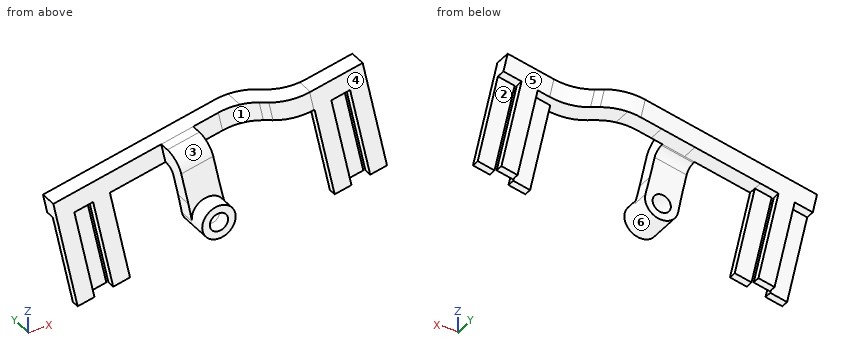
```python
from build123d import *

# Parameters (mm, degrees)
SKETCH1_R             = 3.175
BOSS_EXTRUDE1_DEPTH   = 8.89
F_4_CLEARANCE_HOLE1_D = 3.4544
BOSS_EXTRUDE2_START   = -3.175
BOSS_EXTRUDE2_DEPTH   = 3.175
BOSS_EXTRUDE3_DEPTH   = 3.81
BOSS_EXTRUDE4_START   = -9.525
BOSS_EXTRUDE4_DEPTH   = 3.175
CUT_EXTRUDE1_DEPTH    = 18.185920344
CUT_EXTRUDE2_DEPTH    = 5.08
BOSS_EXTRUDE5_START   = -20.938172
BOSS_EXTRUDE5_DEPTH   = 6.208698
BOSS_EXTRUDE6_DEPTH   = 3.175
FILLET2_R             = 8.89
FILLET3_R             = 1.5875
FILLET4_R             = 3.175
SKETCH16_R            = 3.175
SKETCH16_R_2          = 1.7272
BOSS_EXTRUDE7_DEPTH   = 2.54


with BuildPart() as part:
    # Sketch1 → Boss-Extrude1 (new body)
    with BuildSketch(Plane(origin=(0, 0, 0), x_dir=(1, 0, 0), z_dir=(0, 1, 0))):
        with Locations(Location((0, 0, 0), (0, 0, 270))):
            Circle(SKETCH1_R)
    extrude(amount=BOSS_EXTRUDE1_DEPTH)

    # #4 Clearance Hole1 (through all)
    with Locations(Plane(origin=(0, 8.89, 0), x_dir=(1, 0, 0), z_dir=(0, 1, 0))):
        with Locations((0, 0)):
            Hole(F_4_CLEARANCE_HOLE1_D / 2)

    # Sketch5 → Boss-Extrude2 (add)
    with BuildSketch(Plane(origin=(0, 8.89, 0), x_dir=(1, 0, 0), z_dir=(0, 1, 0)).offset(BOSS_EXTRUDE2_START)):
        with BuildLine():
            Line((-26.325590973, -8.090556636), (8.584422353, -15.580785179))
            Line((8.584422353, -15.580785179), (9.383698549, -11.85556605))
            Line((9.383698549, -11.85556605), (3.175, -10.523439056))
            Line((3.175, -10.523439056), (3.175, 0))
            ThreePointArc((3.175, 0), (0, -3.175), (-3.175, 0))
            Line((-3.175, 0), (-3.175, -9.160994683))
            Line((-3.175, -9.160994683), (-15.592397098, -6.496740696))
            Line((-15.592397098, -6.496740696), (-11.777286014, 11.284502966))
            Line((-11.777286014, 11.284502966), (-21.711203692, 13.415906155))
            Line((-21.711203692, 13.415906155), (-26.325590973, -8.090556636))
        make_face()
    extrude(amount=BOSS_EXTRUDE2_DEPTH)

    # Sketch11 → Boss-Extrude3 (add)
    with BuildSketch(Plane(origin=(-2.818068695, 0, 13.134287577), x_dir=(0.977747803012258, 0, 0.20978377845940036), z_dir=(-0.20978377845940033, 0, 0.9777478030122579))):
        Polygon((11.661996082, 8.89), (12.977124143, 8.89), (19.327124143, 2.54), (21.821996082, 2.54), (21.821996082, -0.635), (18.011996082, -0.635), (11.661996082, 5.715), align=None)
    extrude(amount=-BOSS_EXTRUDE3_DEPTH)

    # Sketch12 → Boss-Extrude4 (add)
    with BuildSketch(Plane(origin=(0, 8.89, 0), x_dir=(1, 0, 0), z_dir=(0, 1, 0)).offset(BOSS_EXTRUDE4_START)):
        Polygon((18.518340032, -17.712188368), (23.132727312, 3.794274423), (33.066644991, 1.662871234), (28.45225771, -19.843591557), align=None)
    extrude(amount=BOSS_EXTRUDE4_DEPTH)

    # Sketch6 → Cut-Extrude1 (cut)
    with BuildSketch(Plane(origin=(1.796318586, 0, -8.372175215), x_dir=(-0.977747803012258, 0, -0.20978377845940016), z_dir=(0.20978377845940016, 0, -0.977747803012258))):
        Polygon((17.142187862, 7.1755), (17.142187862, 5.715), (20.782854529, 5.715), (20.782854529, 7.1755), (24.042521196, 7.1755), (24.042521196, 8.89), (20.528854529, 8.89), (20.528854529, 7.4295), (17.396187862, 7.4295), (17.396187862, 8.89), (13.882521196, 8.89), (13.882521196, 7.1755), align=None)
        Polygon((-28.722329416, 0.8255), (-28.722329416, -0.635), (-25.081662749, -0.635), (-25.081662749, 0.8255), (-21.821996082, 0.8255), (-21.821996082, 2.54), (-25.335662749, 2.54), (-25.335662749, 1.0795), (-28.468329416, 1.0795), (-28.468329416, 2.54), (-31.981996082, 2.54), (-31.981996082, 0.8255), align=None)
    extrude(amount=-CUT_EXTRUDE1_DEPTH, mode=Mode.SUBTRACT)

    # Sketch13 → Cut-Extrude2 (cut)
    with BuildSketch(Plane(origin=(0, 8.89, 0), x_dir=(1, 0, 0), z_dir=(0, 1, 0))):
        Polygon((-3.175, -9.160994683), (3.175, -10.523439056), (3.175, 7.256560944), (-3.175, 7.256560944), align=None)
    extrude(amount=-CUT_EXTRUDE2_DEPTH, mode=Mode.SUBTRACT)


with BuildPart() as cut_extrude2_piece_1:
    # of the separate pieces the step leaves, piece 1, a body of its own (cut_extrude2_pieces)
    add(part.part.solids().sort_by_distance((-18.52407177, 5.715, -12.732080965))[0])

    # Sketch14 → Boss-Extrude5 (add)
    with BuildSketch(Plane(origin=(-23.507522278, 0, -5.04373094), x_dir=(-0.20978377845940016, 0, 0.977747803012258), z_dir=(-0.977747803012258, 0, -0.20978377845940016)).offset(BOSS_EXTRUDE5_START)):
        Polygon((3.81, 0.635), (13.433205921, 0.635), (13.433205921, 5.715), (9.635481661, 5.715), (9.623205921, 5.715), (9.623205921, 3.81), (3.81, 3.81), align=None)
    extrude(amount=-BOSS_EXTRUDE5_DEPTH)



with BuildPart() as cut_extrude2_piece_2:
    # of the separate pieces the step leaves, piece 2, a body of its own (cut_extrude2_pieces)
    add(part.part.solids().sort_by_distance((0, 0, 3.175))[0])


with BuildPart() as cut_extrude2_piece_1_1:
    add(cut_extrude2_piece_1.part)

    add(cut_extrude2_piece_2.part)  # Boss-Extrude6 merges Cut-Extrude2 piece 2
    # Sketch15 → Boss-Extrude6 (add)
    with BuildSketch(Plane(origin=(0, 3.81, 0), x_dir=(1, 0, 0), z_dir=(0, 1, 0))):
        with BuildLine():
            Line((-3.834546879, -3.073977009), (-3.116253173, 0.607940096))
            ThreePointArc((-3.116253173, 0.607940096), (-0.666063497, -3.104349275), (3.091361375, -0.723954316))
            Line((3.091361375, -0.723954316), (2.235994487, -4.37646125))
            Line((2.235994487, -4.37646125), (-3.834546879, -3.073977009))
        make_face()
    extrude(amount=-BOSS_EXTRUDE6_DEPTH)

    # Fillet2
    fillet2_edges = [cut_extrude2_piece_1_1.edges().sort_by_distance(p)[0] for p in [
        (8.984060451, 5.715, 13.718175614),
        (10.269924023, 8.89, 13.994068148),
        (16.478622572, 2.54, 15.326195141),
        (15.192759, -0.635, 15.050302607),
    ]]
    fillet(fillet2_edges, radius=FILLET2_R)

    # Fillet3
    fillet3_edges = [cut_extrude2_piece_1_1.edges().sort_by_distance(p)[0] for p in [
        (-2.01879269, 3.81, 9.409068406),
    ]]
    fillet(fillet3_edges, radius=FILLET3_R)

    # Fillet4
    fillet4_edges = [cut_extrude2_piece_1_1.edges().sort_by_distance(p)[0] for p in [
        (-2.818068886, 0.635, 13.134287535),
    ]]
    fillet(fillet4_edges, radius=FILLET4_R)

    # Sketch16 → Boss-Extrude7 (add)
    with BuildSketch(Plane.XZ):
        with Locations(Location((0, 0, 0), (0, 0, 270))):
            Circle(SKETCH16_R)
        with Locations(Location((0, 0, 0), (0, 0, 270))):
            Circle(SKETCH16_R_2, mode=Mode.SUBTRACT)
    extrude(amount=BOSS_EXTRUDE7_DEPTH)


solid = cut_extrude2_piece_1_1.part
```
The model under review builds one solid part; all positions refer to its coordinate system, in mm. Face numbers are marked on the shaded views. A direction names the side the tool comes from. Round coordinates to 2 decimals unless told otherwise and drop trailing zeros. Loops run counter-clockwise (first coordinate to the right, second up) from the corner with the lowest first, then second, coordinate; pieces in that order, holes last. Notation, with made-up numbers: (33.25, -13) - (90.25, -13) arc R11 ccw to (90.25, -6) - close; hole circle Ø2 at (81.5, 51). An arc over 180 degrees is marked (long way). Write each question's results on one line, items separated by ' | '. Start each with the question number.
Q1. Insertion check: P1, Ø10, axis at x = 19.5, z = 7.5, coming from the -Y side (3 decimals); P2, Ø8, axis at x = 24, z = 10.5, coming from the +Y side; P3, Ø5.5, axis at x = -23, z = -5.5, coming from the +Y side; P4, Ø4.5, axis at x = 0, z = 0, coming from the -Y side. Each pin has a flat end and moves straight along its axis. Give the tip position at first contact, or say it passes through.
Q2. Wall thickness on line 1 along X through (y, z) = (-0.9, 0) (3 decimals); line 2 along X through (y, z) = (1.25, 0.5); line 3 along Z through (x, y) = (0, 2.2) (3 decimals): over which ranges is each line inside the solid? List them lowest first. Write a range as [from, to].
Q3. Take a section at C-C on y = 8. Give the boundary of the cut face in (x, z) (3 decimals), plus the area to 3 significant figures.
Q4. Tool access review of the marked faces 4, 5 and 6: name each direction out of +Z, -Z, +X, -X, +Y, -Y from which nothing blocks a thin tool from reaching the whole face with its end or side.
Q5. Take a section at B-B on z = 0. Give the number of separate pieces and of enclosed holes in the cut face, plus the area to 3 significant figures.
Q6. Take a section at A-A on z = -6. Give the boundary of the cut face in (x, y) (1 decimal).
Q7. Draft analysis for pull direction X (two halves, no side actions). For the marked faces 1, 2 and 3, state which applies: pulls with the +X half, pulls with the -X half, needs draft (parallel to the pull), parting line crosses it, or undercut.
Data:
1) P1: stops at y = -0.635 | P2: stops at y = 2.54 | P3: stops at y = 7.18 | P4: stops at y = -2.54
2) line 1: x = [-3.175, -1.727], [1.727, 3.175] | line 2: x = [-3.33, -1.65], [1.65, 3.14], [25.8, 29.01] | line 3: z = [-3.175, -1.727], [1.727, 13.29]
3) outline: (-26.326, 8.091) - (-25.526, 4.365) - (-22.091, 5.102) - (-18.276, -12.679) - (-15.213, -12.022) - (-19.028, 5.76) - (10.86, 12.172) - (10.061, 15.898) - close | area: 199 mm²
4) face 4: +Z, -Z, +X, -Y | face 5: +Z, -Z, +X, +Y | face 6: -Y
5) separate pieces: 8 | enclosed holes: 0 | area: 47.4 mm²
6) outline: (-23.3, 5.7) - (-20, 5.7) - (-20, 7.2) - (-23.3, 7.2) - close; (-19.7, 7.4) - (-16.5, 7.4) - (-16.5, 8.9) - (-19.7, 8.9) - close; (-16.2, 5.7) - (-12.9, 5.7) - (-12.9, 7.2) - (-16.2, 7.2) - close
7) face 1: undercut | face 2: needs draft | face 3: pulls with the -X half
